from build123d import *

# Parameters (mm, degrees)
SKETCH1_R           = 37.465
BOSS_EXTRUDE1_DEPTH = 57.15
BOSS_EXTRUDE2_START = 69.85
SKETCH1_3_R         = 76.2
SKETCH1_3_R_2       = 57.15
SKETCH1_3_R_3       = 37.465
BOSS_EXTRUDE2_DEPTH = 12.7
BOSS_EXTRUDE3_START = 133.35
SKETCH1_4_R         = 57.15
SKETCH1_4_R_2       = 37.465
BOSS_EXTRUDE3_DEPTH = 63.5
BOSS_EXTRUDE4_START = -57.15
SKETCH1_5_R         = 76.2
SKETCH1_5_R_2       = 57.15
SKETCH1_5_R_3       = 37.465
BOSS_EXTRUDE4_DEPTH = 12.7
BOSS_EXTRUDE5_START = -69.85
SKETCH1_6_R         = 57.15
SKETCH1_6_R_2       = 37.465
BOSS_EXTRUDE5_DEPTH = 63.5


with BuildPart() as part:
    # Sketch1 → Boss-Extrude1 (new, symmetric)
    with BuildSketch(Plane(origin=(0, 0, 0), x_dir=(0, 0, -1), z_dir=(1, 0, 0))):
        Circle(SKETCH1_R)
    extrude(amount=BOSS_EXTRUDE1_DEPTH, both=True)

    # Sketch1<3> → Boss-Extrude2 (add)
    # profile 1 of 3: a face of its own
    with BuildSketch(Plane(origin=(0, 0, 0), x_dir=(0, 0, -1), z_dir=(1, 0, 0)).offset(BOSS_EXTRUDE2_START)):
        Circle(SKETCH1_3_R)
        Circle(SKETCH1_3_R_2, mode=Mode.SUBTRACT)
    # profile 2 of 3: a face of its own
    with BuildSketch(Plane(origin=(0, 0, 0), x_dir=(0, 0, -1), z_dir=(1, 0, 0)).offset(BOSS_EXTRUDE2_START)):
        Circle(SKETCH1_3_R_2)
        Circle(SKETCH1_3_R_3, mode=Mode.SUBTRACT)
    # profile 3 of 3: a face of its own
    with BuildSketch(Plane(origin=(0, 0, 0), x_dir=(0, 0, -1), z_dir=(1, 0, 0)).offset(BOSS_EXTRUDE2_START)):
        Circle(SKETCH1_3_R_3)
    extrude(amount=-BOSS_EXTRUDE2_DEPTH)

    # Sketch1<4> → Boss-Extrude3 (add)
    # profile 1 of 2: a face of its own
    with BuildSketch(Plane(origin=(0, 0, 0), x_dir=(0, 0, -1), z_dir=(1, 0, 0)).offset(BOSS_EXTRUDE3_START)):
        Circle(SKETCH1_4_R)
        Circle(SKETCH1_4_R_2, mode=Mode.SUBTRACT)
    # profile 2 of 2: a face of its own
    with BuildSketch(Plane(origin=(0, 0, 0), x_dir=(0, 0, -1), z_dir=(1, 0, 0)).offset(BOSS_EXTRUDE3_START)):
        Circle(SKETCH1_4_R_2)
    extrude(amount=-BOSS_EXTRUDE3_DEPTH)

    # Sketch1<5> → Boss-Extrude4 (add)
    # profile 1 of 3: a face of its own
    with BuildSketch(Plane(origin=(0, 0, 0), x_dir=(0, 0, -1), z_dir=(1, 0, 0)).offset(BOSS_EXTRUDE4_START)):
        Circle(SKETCH1_5_R)
        Circle(SKETCH1_5_R_2, mode=Mode.SUBTRACT)
    # profile 2 of 3: a face of its own
    with BuildSketch(Plane(origin=(0, 0, 0), x_dir=(0, 0, -1), z_dir=(1, 0, 0)).offset(BOSS_EXTRUDE4_START)):
        Circle(SKETCH1_5_R_2)
        Circle(SKETCH1_5_R_3, mode=Mode.SUBTRACT)
    # profile 3 of 3: a face of its own
    with BuildSketch(Plane(origin=(0, 0, 0), x_dir=(0, 0, -1), z_dir=(1, 0, 0)).offset(BOSS_EXTRUDE4_START)):
        Circle(SKETCH1_5_R_3)
    extrude(amount=-BOSS_EXTRUDE4_DEPTH)

    # Sketch1<6> → Boss-Extrude5 (add)
    # profile 1 of 2: a face of its own
    with BuildSketch(Plane(origin=(0, 0, 0), x_dir=(0, 0, -1), z_dir=(1, 0, 0)).offset(BOSS_EXTRUDE5_START)):
        Circle(SKETCH1_6_R)
        Circle(SKETCH1_6_R_2, mode=Mode.SUBTRACT)
    # profile 2 of 2: a face of its own
    with BuildSketch(Plane(origin=(0, 0, 0), x_dir=(0, 0, -1), z_dir=(1, 0, 0)).offset(BOSS_EXTRUDE5_START)):
        Circle(SKETCH1_6_R_2)
    extrude(amount=-BOSS_EXTRUDE5_DEPTH)


solid = part.part
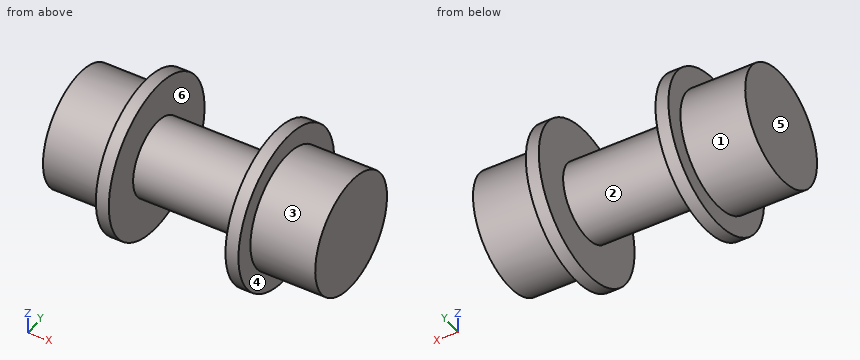
Can you work these out from the model? Positions are in its coordinate system, mm. Face numbers are marked on the shaded views. A direction names the side the tool comes from. Coordinates: 2 decimals unless noted, no trailing zeros. Order: outer loops, then holes, each group sorted by start corner. A loop starts at its lowest first (then second) coordinate and runs counter-clockwise, first axis right, second up. Notation, with made-up numbers: (42.5, 15) - (73.5, 15) arc R30 ccw to (73.5, 49) - close; hole circle Ø6 at (8.25, -9). An arc over 180 degrees is marked (long way). Answer as a JSON object with one key per item and string values. Group by question number.
Q1. Will these pins go through, and if not, where does the flat tip stop? P1, Ø12, axis at x = 65.5, y = -39.5, coming from the -Z side; P2, Ø3, axis at x = 10.5, y = 30, coming from the +Z side; P3, Ø1.5, axis at y = 56, z = 30, coming from the +X side.
Q2. Imagine slicing it at C-C (z = -63.5). Please give me the cut outline in (x, y).
Q3. Imagine slicing it at A-A (z = 0). Please give me the cut outline in (x, y) (3 decimals), and give its area (3 significant figures).
Q4. We'd pull the mould along X, two halves only. Please class the marked faces 4, 5 and 6: +X half, -X half, draft (parallel to the pull), parting line (faces both ways), or undercut.
Q5. I need wall thicknesses on line 1 (X direction, y = -59, z = 12.5); line 2 (X direction, y = 36.5, z = 38); line 3 (Y direction, x = -30.5, z = 26). Which ranges of each line are inside material? Lowest first, please. Write a range as from..to.
Q6. Imagine slicing it at B-B (y = -48). Please give me the cut outline in (x, z), and give its area (3 significant figures).
Q7. On a 3-axis mill with a long thin cutter (end or side, diameter ignored), from which of +Z, -Z, +X, -X, +Y, -Y can I reach the whole of each face in a straight line? I mean the marked faces 1, 2 and 3. Say none if no direction works.
Determined:
{
 "1": {"P1": "stops at z = -68.44", "P2": "stops at z = 24.32", "P3": "stops at x = 69.85"},
 "2": {"outline": "(-69.85, -42.12) - (-57.15, -42.12) - (-57.15, 42.12) - (-69.85, 42.12) - close; (57.15, -42.12) - (69.85, -42.12) - (69.85, 42.12) - (57.15, 42.12) - close"},
 "3": {"outline": "(-133.35, -57.15) - (-69.85, -57.15) - (-69.85, -76.2) - (-57.15, -76.2) - (-57.15, -37.465) - (57.15, -37.465) - (57.15, -76.2) - (69.85, -76.2) - (69.85, -57.15) - (133.35, -57.15) - (133.35, 57.15) - (69.85, 57.15) - (69.85, 76.2) - (57.15, 76.2) - (57.15, 37.465) - (-57.15, 37.465) - (-57.15, 76.2) - (-69.85, 76.2) - (-69.85, 57.15) - (-133.35, 57.15) - close", "area": "27,000 mm2"},
 "4": {"face 4": "+X half", "face 5": "-X half", "face 6": "undercut"},
 "5": {"line 1": "x = -69.85..-57.15, 57.15..69.85", "line 2": "x = -133.35..-57.15, 57.15..133.35", "line 3": "y = -26.97..26.97"},
 "6": {"outline": "(-133.35, -31.02) - (-69.85, -31.02) - (-69.85, -59.18) - (-57.15, -59.18) - (-57.15, 59.18) - (-69.85, 59.18) - (-69.85, 31.02) - (-133.35, 31.02) - close; (57.15, -59.18) - (69.85, -59.18) - (69.85, -31.02) - (133.35, -31.02) - (133.35, 31.02) - (69.85, 31.02) - (69.85, 59.18) - (57.15, 59.18) - close", "area": "10,900 mm2"},
 "7": {"face 1": "-X", "face 2": "none", "face 3": "+X"}
}
